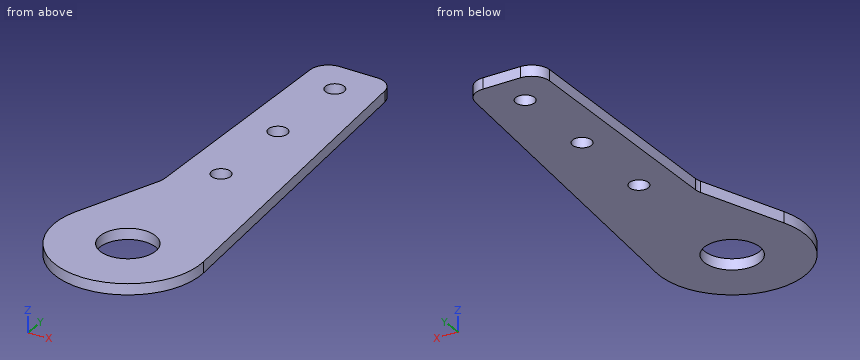
from build123d import *

# Parameters (mm, degrees)
SKETCH_2_R      = 7.6
SKETCH_2_R_2    = 2.6
EXTRUDE_1_DEPTH = 3
FILLET_7_R      = 5


with BuildPart() as part:
    # ｽｹｯﾁ2 → ﾎﾞｽ - 押し出し1 (new body)
    with BuildSketch(Plane.XY):
        with BuildLine():
            Line((-10, 101), (-10, 31))
            Line((-10, 31), (-18.793732859, 6.840731336))
            ThreePointArc((-18.793732859, 6.840731336), (-2.487711667, -19.844679152), (19.900748755, 1.990024876))
            Line((19.900748755, 1.990024876), (10, 101))
            Line((10, 101), (-10, 101))
        make_face()
        Circle(SKETCH_2_R, mode=Mode.SUBTRACT)
        with Locations((0, 66)):
            Circle(SKETCH_2_R_2, mode=Mode.SUBTRACT)
        with Locations((0, 91)):
            Circle(SKETCH_2_R_2, mode=Mode.SUBTRACT)
        with Locations((0, 41)):
            Circle(SKETCH_2_R_2, mode=Mode.SUBTRACT)
    extrude(amount=EXTRUDE_1_DEPTH)

    # ﾌｨﾚｯﾄ7
    fillet_7_edges = [part.edges().sort_by_distance(p)[0] for p in [
        (10, 101, 1.5),
        (-10, 31, 1.5),
        (-10, 101, 1.5),
    ]]
    fillet(fillet_7_edges, radius=FILLET_7_R)


solid = part.part
Geometry: final body of the model. Coordinates: model frame, mm. Give positions to 0.01 mm unless a question says otherwise; leave off trailing zeros. Loops run counter-clockwise (first coordinate to the right, second up) from the corner with the lowest first, then second, coordinate; pieces in that order, holes last. Notation, with made-up numbers: M 80,-29 L 118,-29 A26 ccw 118,-11 Z; hole C 14.25,48.25 d11. An arc over 180 degrees is marked long. Put each result on its own line as item: value. Start each with the question number.
1) Cut plane C-C (z = 1.3). Output: boundary loops of the cut face in (x, y).
2) Cut plane B-B (y = 0). Output: boundary loops of the cut face in (x, z).
3) Ray query, line 1 along Y through (x, z) = (0, 1.25); line 2 along Y through (x, z) = (1, 1.45); line 3 along X through (y, z) = (40.5, 1.35). Return the intervals inside material, ascending.
4) Cut plane D-D (y = 41). Output: boundary loops of the cut face in (x, z), then the cut area to 3 significant figures.
5) Cut plane A-A (x = 0). Output: boundary loops of the cut face in (y, z), then the cut area to 3 significant figures.
6) Contact query for flat-ended pins moving along their axis: pin 1 (1.5 mm diameter, centred on y = 53.5, z = 1.5, fed in from -X); pin 2 (12 mm diameter, centred on x = -4.5, y = 4.5, fed in from -Z). Output: stop coordinate, or through.
Verdict:
1. outline: M -18.79,6.84 A20 ccw long 19.9,1.99 L 10.45,96.5 A5 ccw 5.48,101 L -5,101 A5 ccw -10,96 L -10,31.88 A5 cw -10.3,30.17 Z; hole C 0,0 d15.2; hole C 0,41 d5.2; hole C 0,66 d5.2; hole C 0,91 d5.2
2. outline: M -20,0 L -7.6,0 L -7.6,3 L -20,3 Z; M 7.6,0 L 20,0 L 20,3 L 7.6,3 Z
3. line 1: -20 to -7.6, 7.6 to 38.4, 43.6 to 63.4, 68.6 to 88.4, 93.6 to 101
3. line 2: -19.97 to -7.53, 7.53 to 38.6, 43.4 to 63.6, 68.4 to 88.6, 93.4 to 101
3. line 3: -10 to -2.55, 2.55 to 16.05
4. outline: M -10,0 L -2.6,0 L -2.6,3 L -10,3 Z; M 2.6,0 L 16,0 L 16,3 L 2.6,3 Z
4. area: 62.4 mm2
5. outline: M -20,0 L -7.6,0 L -7.6,3 L -20,3 Z; M 7.6,0 L 38.4,0 L 38.4,3 L 7.6,3 Z; M 43.6,0 L 63.4,0 L 63.4,3 L 43.6,3 Z; M 68.6,0 L 88.4,0 L 88.4,3 L 68.6,3 Z; M 93.6,0 L 101,0 L 101,3 L 93.6,3 Z
5. area: 271 mm2
6. pin 1: x = -10
6. pin 2: z = 0
